```python
from build123d import *

# Parameters (mm, degrees)
SKETCH2_W           = 177.8
SKETCH2_H           = 101.6
BOSS_EXTRUDE3_DEPTH = 6.35
SKETCH3_W           = 6.35
SKETCH3_H           = 12.895827841
SKETCH3_W_2         = 67.9
SKETCH3_H_2         = 25.4
SKETCH3_H_3         = 12.7
SKETCH3_W_3         = 49.509
SKETCH3_W_4         = 18.391
CUT_EXTRUDE3_DEPTH  = 103.587389576
SKETCH4_W           = 44.937577928
SKETCH4_H           = 11.22448853
SKETCH4_W_2         = 5.08
SKETCH4_H_2         = 63.5
CUT_EXTRUDE4_DEPTH  = 103.587389576
SKETCH5_W           = 3
SKETCH5_H           = 5
CUT_EXTRUDE5_DEPTH  = 103.587389576


with BuildPart() as part:
    # Sketch2 → Boss-Extrude3 (new body)
    with BuildSketch(Plane.XY):
        Rectangle(SKETCH2_W, SKETCH2_H)
    extrude(amount=BOSS_EXTRUDE3_DEPTH)

    # Sketch3 → Cut-Extrude3 (cut, through all)
    with BuildSketch(Plane.XY.offset(6.35)):
        with Locations((-85.725, 18.95208608)):
            Rectangle(SKETCH3_W, SKETCH3_H)
        with Locations((-40.95, 38.1)):
            Rectangle(SKETCH3_W_2, SKETCH3_H_2)
        with Locations((-85.725, -19.05)):
            Rectangle(SKETCH3_W, SKETCH3_H_3)
        with Locations((31.7545, 38.1)):
            Rectangle(SKETCH3_W_3, SKETCH3_H_2)
        with Locations((79.7045, 38.1)):
            Rectangle(SKETCH3_W_4, SKETCH3_H_2)
        with Locations((-40.95, -44.45)):
            Rectangle(SKETCH3_W_2, SKETCH3_H_3)
        with Locations((31.7545, -44.45)):
            Rectangle(SKETCH3_W_3, SKETCH3_H_3)
        with Locations((79.7045, -44.45)):
            Rectangle(SKETCH3_W_4, SKETCH3_H_3)
    extrude(amount=-CUT_EXTRUDE3_DEPTH, mode=Mode.SUBTRACT)

    # Sketch4 → Cut-Extrude4 (cut, through all)
    with BuildSketch(Plane(origin=(0, 0, 0), x_dir=(-1, 0, 0), z_dir=(0, 0, -1))):
        with Locations((40.95, 19.787755735)):
            Rectangle(SKETCH4_W, SKETCH4_H)
        with Locations((-86.36, -6.35)):
            Rectangle(SKETCH4_W_2, SKETCH4_H_2)
        Polygon((-17.768385345, 25.4), (-31.7545, 25.4), (-45.740614655, 25.4), (-45.740614655, 14.176), (-17.768385345, 14.176), align=None)
    extrude(amount=-CUT_EXTRUDE4_DEPTH, mode=Mode.SUBTRACT)

    # Sketch5 → Cut-Extrude5 (cut, through all)
    with BuildSketch(Plane(origin=(0, 0, 0), x_dir=(-1, 0, 0), z_dir=(0, 0, -1))):
        with Locations((-28.6295, -9.35)):
            Rectangle(SKETCH5_W, SKETCH5_H)
        with Locations((-34.8795, -9.35)):
            Rectangle(SKETCH5_W, SKETCH5_H)
    extrude(amount=-CUT_EXTRUDE5_DEPTH, mode=Mode.SUBTRACT)


solid = part.part
```
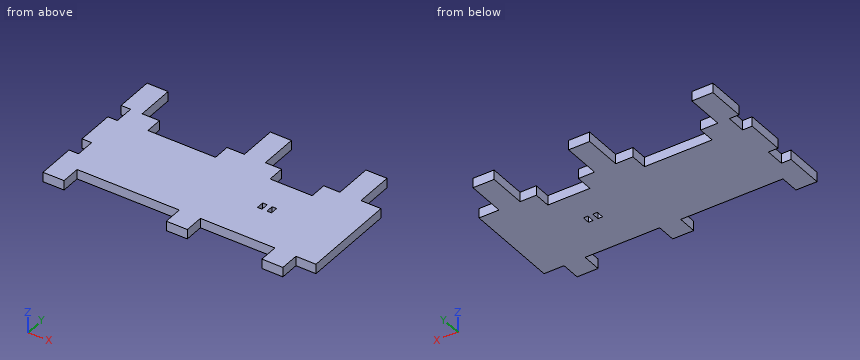
Here's how the part is built. I have some questions about the finished solid (model axes, mm). Round coordinates to 2 decimals unless told otherwise and drop trailing zeros. Write each loop counter-clockwise with the first axis right and the second up, starting at its lowest first coordinate (ties: lowest second). Pieces come first, ordered by that corner, then holes.
Q1. Please list where these lines run through material, in increasing order: probe 1 along X at (y, z) = (27, 0.75); probe 2 along X at (y, z) = (22, 1.25); probe 3 along Y at (x, z) = (-67, 5.75).
Q2. If we section it at A-A on y = 37.5: Write out the boundary of the cut face in (x, z).
Q3. If we section it at B-B on z = 3.75: Give the number of separate pieces and of enclosed holes in the cut face, plus the area to 3 significant figures.
Q4. Will these pins go through, and if not, where does the flat tip stop? P1, Ø3, axis at x = 51.5, z = 3, coming from the +Y side; P2, Ø3, axis at y = 22, z = 4, coming from the -X side; P3, Ø3, axis at y = -46.5, z = 2, coming from the +X side.
Q5. If we section it at D-D on x = 72.5: Write out the boundary of the cut face in (y, z).
Q6. If we section it at C-C on x = -42: Write out the boundary of the cut face in (y, z).
Answer below:
1. probe 1: x = -88.9 to -74.9, -7 to 7, 56.51 to 70.51
1. probe 2: x = -82.55 to -63.42, -18.48 to 17.77, 45.74 to 83.82
1. probe 3: y = -38.1 to 25.4
2. outline: (-88.9, 0) - (-74.9, 0) - (-74.9, 6.35) - (-88.9, 6.35) - close; (-7, 0) - (7, 0) - (7, 6.35) - (-7, 6.35) - close; (56.51, 0) - (70.51, 0) - (70.51, 6.35) - (56.51, 6.35) - close
3. separate pieces: 1
3. enclosed holes: 2
3. area: 11,600 mm2
4. P1: stops at y = 25.4
4. P2: stops at x = -82.55
4. P3: stops at x = 70.51
5. outline: (-38.1, 0) - (25.4, 0) - (25.4, 6.35) - (-38.1, 6.35) - close
6. outline: (-38.1, 0) - (14.18, 0) - (14.18, 6.35) - (-38.1, 6.35) - close
